Could you check a few things on this drawing? It's one solid part, dimensions in mm from its lowest x, y, z. A direction names the side the tool comes from. Round coordinates to 2 decimals unless told otherwise and drop trailing zeros. Loops run counter-clockwise (first coordinate to the right, second up) from the corner with the lowest first, then second, coordinate; pieces in that order, holes last. Notation, with made-up numbers: M 82.5,70 L 100.5,70 A20 cw 100.5,88 Z; hole C 26.25,41 d11. An arc over 180 degrees is marked long. Return JSON: item names as keys, results as strings.
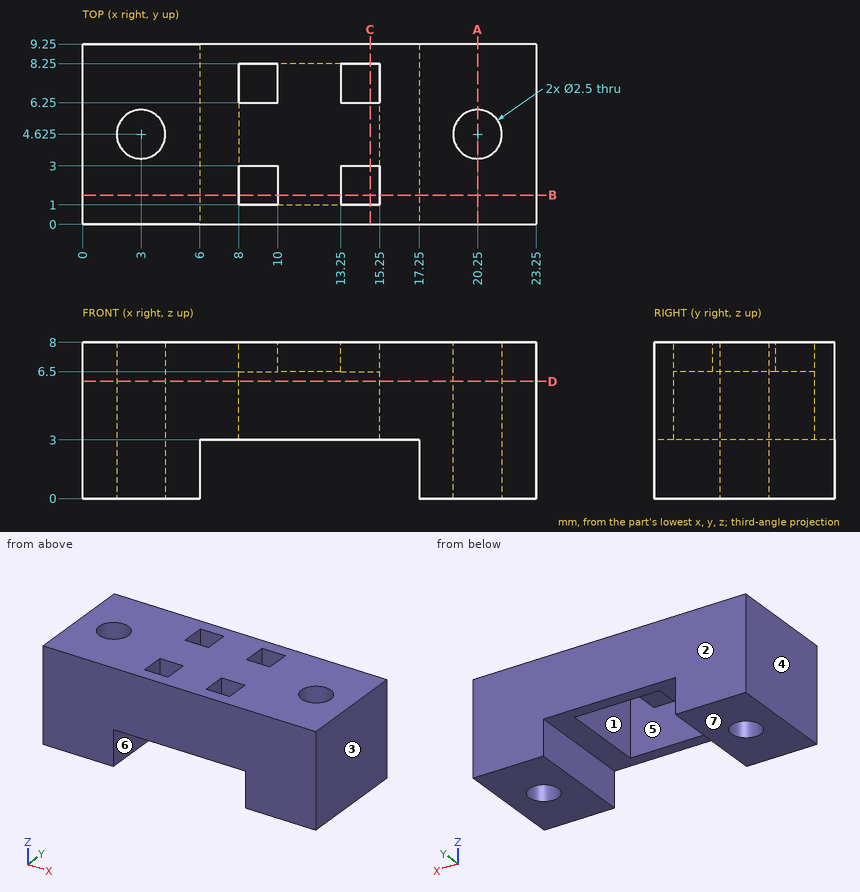
Q1. Suppose I cut it at A-A, the plane x = 20.25. Please give me the cut outline in (y, z) (3 decimals).
Results:
{"outline": "M 0,0 L 3.375,0 L 3.375,8 L 0,8 Z; M 5.875,0 L 9.25,0 L 9.25,8 L 5.875,8 Z"}
Q2. If I drill on line 1 along X through (y, z) = (2.75, 2.75); line 2 along Y through (x, z) = (3, 5) (3 decimals); line 3 along X through (y, z) = (4.25, 4.75), over which ranges is the centre line in solid material (lowest first)?
Results:
{"line 1": "x = 0 to 6, 17.25 to 23.25", "line 2": "y = 0 to 3.375, 5.875 to 9.25", "line 3": "x = 0 to 1.81, 4.19 to 8, 15.25 to 19.06, 21.44 to 23.25"}
Q3. On a 3-axis mill with a long thin cutter (end or side, diameter ignored), from which of +Z, -Z, +X, -X, +Y, -Y can I reach the whole of each face in a straight line? I mean the marked faces 5, 6 and 7. Say none if no direction works.
Results:
{"face 5": "-Z", "face 6": "-Z, +Y, -Y", "face 7": "-Z, +X, -X, +Y, -Y"}
Q4. Thinking about a two-plate mould opening in X: for the marked faces 1, 2, 3 and 4, which applies, pulls with the +X half, pulls with the -X half, needs draft (parallel to the pull), parting line crosses it, or undercut?
Results:
{"face 1": "undercut", "face 2": "needs draft", "face 3": "pulls with the +X half", "face 4": "pulls with the -X half"}
Q5. Suppose I cut it at D-D, the plane z = 6. Please give me the cut outline in (x, y) (3 decimals), plus the area to 3 significant figures.
Results:
{"outline": "M 0,0 L 23.25,0 L 23.25,9.25 L 0,9.25 Z; hole C 3,4.625 d2.5; hole M 8,1 L 15.25,1 L 15.25,8.25 L 8,8.25 Z; hole C 20.25,4.625 d2.5", "area": "153 mm2"}
Q6. Suppose I cut it at C-C, the plane x = 14.75. Please give me the cut outline in (y, z).
Results:
{"outline": "M 0,3 L 1,3 L 1,8 L 0,8 Z; M 3,6.5 L 6.25,6.5 L 6.25,8 L 3,8 Z; M 8.25,3 L 9.25,3 L 9.25,8 L 8.25,8 Z"}
Q7. Suppose I cut it at B-B, the plane y = 1.5. Please give me the cut outline in (x, z), plus the area to 3 significant figures.
Results:
{"outline": "M 0,0 L 6,0 L 6,3 L 8,3 L 8,8 L 0,8 Z; M 10,6.5 L 13.25,6.5 L 13.25,8 L 10,8 Z; M 15.25,3 L 17.25,3 L 17.25,0 L 23.25,0 L 23.25,8 L 15.25,8 Z", "area": "121 mm2"}
